For this review, take the finished solid that the model builds, in its own axes (mm). Face numbers are marked on the shaded views. Round coordinates to 2 decimals unless told otherwise and drop trailing zeros. Loops run counter-clockwise (first coordinate to the right, second up) from the corner with the lowest first, then second, coordinate; pieces in that order, holes last.
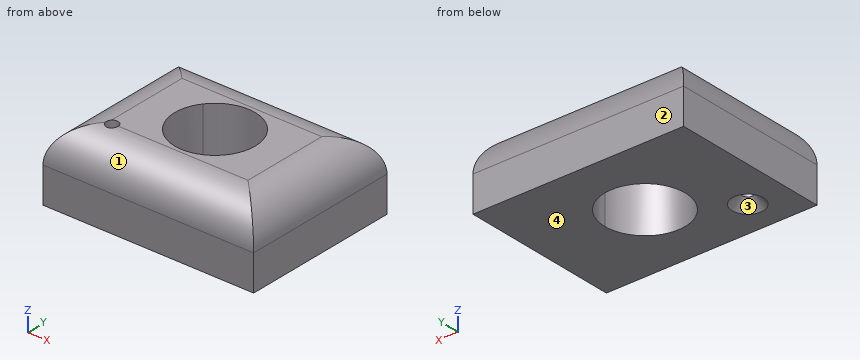
```python
from build123d import *

# Parameters (mm, degrees)
F0_W           = 75.4651799798
F0_H           = 56.8607151508
F1_DEPTH       = 25.4
F2_R           = 12.7
F4_D           = 4.2
F4_CSINK_D     = 11.2
F4_CSINK_ANGLE = 90


with BuildPart() as f1:
    # F0 (on Top) → F1 (new body)
    with BuildSketch(Plane.XY):
        Rectangle(F0_W, F0_H)
        with BuildLine():
            ThreePointArc((14.4115838808, 0), (-4.5724943597, -13.6669691331), (-11.5100700927, 8.6724873257))
            ThreePointArc((-11.5100700927, 8.6724873257), (4.5724943597, 13.6669691331), (14.4115838808, 0))
        make_face(mode=Mode.SUBTRACT)
    extrude(amount=F1_DEPTH)

    # F2
    f2_edges = [f1.edges().sort_by_distance(p)[0] for p in [
        (0, -28.430358, 25.4),
        (-37.73259, 0, 25.4),
        (0, 28.430358, 25.4),
        (37.73259, 0, 25.4),
    ]]
    fillet(f2_edges, radius=F2_R)

    # F4 (through all)
    with Locations(Plane(origin=(0, 0, 0), x_dir=(1, 0, 0), z_dir=(0, 0, -1))):
        with Locations((-23.5218573362, 15.828538686)):
            CounterSinkHole(F4_D / 2, F4_CSINK_D / 2, counter_sink_angle=F4_CSINK_ANGLE)


solid = f1.part
```
(1) Add section B-B (y = 1.5). Give the boundary of the cut face in (x, z).
(2) Add section C-C (z = 19.5). Give the boundary of the cut face in (x, y), plus the area to 3 significant figures.
(3) Add section A-A (x = 0). Give the boundary of the cut face in (y, z), plus the area to 3 significant figures.
(4) Insertion check: pin 1 Ø5 at (x, z) = (-27, 20.5) entering from +Y; pin 2 Ø1 at (y, z) = (4, 19) entering from -X; pin 3 Ø6 at (x, y) = (-23.5, -21.5) entering from +Z. Each pin has a flat end and moves straight along its axis. Give the tip position at first contact, or say it passes through.
(5) Add section D-D (x = 18). Give the boundary of the cut face in (y, z).
(6) The part is to be moulded in two halves that separate along Y. For the marked faces 1, 2, 3 and 4, say which applies: pulls with the +Y half, pulls with the -Y half, needs draft (parallel to the pull), parting line crosses it, or undercut.
(7) For L1, parallel to X at y = 0, z = 9.75; L2, parallel to Z at x = -25.5, y = -5; L3, parallel to X at y = 11, z = 15.75, list the stretches that pass through material, from the lowest coordinate up.
Outcome:
1. outline: (-37.73, 0) - (-14.33, 0) - (-14.33, 25.4) - (-25.03, 25.4) arc R12.7 ccw to (-37.73, 12.7) - close; (14.33, 0) - (37.73, 0) - (37.73, 12.7) arc R12.7 ccw to (25.03, 25.4) - (14.33, 25.4) - close
2. outline: (-35.76, -26.46) - (35.76, -26.46) - (35.76, 26.46) - (-35.76, 26.46) - close; hole circle Ø4.2 at (-23.52, -15.83); hole circle Ø28.82 at (0, 0)
2. area: 3,120 mm2
3. outline: (-28.43, 0) - (-14.41, 0) - (-14.41, 25.4) - (-15.73, 25.4) arc R12.7 ccw to (-28.43, 12.7) - close; (14.41, 0) - (28.43, 0) - (28.43, 12.7) arc R12.7 ccw to (15.73, 25.4) - (14.41, 25.4) - close
3. area: 643 mm2
4. pin 1: stops at y = 27.27
4. pin 2: stops at x = -36.33
4. pin 3: stops at z = 25.09
5. outline: (-28.43, 0) - (28.43, 0) - (28.43, 12.7) arc R12.7 ccw to (15.73, 25.4) - (-15.73, 25.4) arc R12.7 ccw to (-28.43, 12.7) - close
6. face 1: pulls with the -Y half
6. face 2: pulls with the +Y half
6. face 3: undercut
6. face 4: needs draft
7. L1: x = -37.73 to -14.41, 14.41 to 37.73
7. L2: z = 0 to 25.39
7. L3: x = -37.36 to -9.31, 9.31 to 37.36
